from build123d import *

# Parameters (mm, degrees)
BOSS_EXTRU_1_DEPTH      = 20
CONG_1_R                = 2.38125
ESQUISSE2_W             = 63.5
ESQUISSE2_H             = 35.56
BOSS_EXTRU_2_DEPTH      = 5.08
EMPREINTE1_START        = -25.08
EMPREINTE1_DEPTH        = 5.08
D_PLACER_START          = -25.08
D_PLACER_LA_FACE1_DEPTH = 5.08
EMPREINTE4_START        = 17.46
EMPREINTE4_DEPTH        = 2.54
D_PLACER_START_2        = 16.952
D_PLACER_LA_FACE2_DEPTH = 3.048
CHANFREIN1_SIZE         = 6.35
CHANFREIN1_SIZE2        = 3.81
CHANFREIN2_SIZE         = 3.81
CHANFREIN2_SIZE2        = 6.35
BOSS_EXTRU_3_DEPTH      = 45.08
ESQUISSE4_W             = 44.45
ESQUISSE4_H             = 27.94
ENL_V_MAT_EXTRU_1_DEPTH = 38.1
ESQUISSE5_W             = 12.7
ESQUISSE5_H             = 3.81
BOSS_EXTRU_4_DEPTH      = 12.7
CONG_2_R                = 2.54
D_GAGEMENT_61_D         = 3.7973
ENL_V_MAT_EXTRU_2_DEPTH = 38.1
D_GAGEMENT_62_D         = 3.7973
D_GAGEMENT_62_DEPTH     = 18.796
D_GAGEMENT_62_TIP       = 1.140824014


# Read off the part's stored shape, not the designer's step: Empreinte1, Déplacer la face1, Empreinte4, Déplacer la face2
with BuildPart() as part:
    # Esquisse1 → Boss.-Extru.1 (new, symmetric)
    with BuildSketch(Plane.XY):
        Polygon((-31.75, -1.905), (-31.75, 33.655), (31.75, 33.655), (31.75, -1.905), (12.92225, -1.905), (12.92225, 4.445), (13.87475, 5.3975), (21.59, 5.3975), (21.59, 21.59), (-21.59, 21.59), (-21.59, 5.3975), (-13.87475, 5.3975), (-12.92225, 4.445), (-12.92225, -1.905), align=None)
    extrude(amount=BOSS_EXTRU_1_DEPTH, both=True)

    # Congé1
    cong_1_edges = [part.edges().sort_by_distance(p)[0] for p in [
        (21.59, 5.3975, 0),
        (21.59, 21.59, 0),
        (-21.59, 21.59, 0),
        (-21.59, 5.3975, 0),
    ]]
    fillet(cong_1_edges, radius=CONG_1_R)

    # Esquisse2 → Boss.-Extru.2 (add)
    with BuildSketch(Plane(origin=(0, 0, -20), x_dir=(-1, 0, 0), z_dir=(0, 0, -1))):
        with Locations((0, 15.875)):
            Rectangle(ESQUISSE2_W, ESQUISSE2_H)
    extrude(amount=BOSS_EXTRU_2_DEPTH)

    # Empreinte1 outline → Empreinte1 (cut)
    with BuildSketch(Plane.XY.offset(EMPREINTE1_START)):
        with BuildLine():
            Line((14.44625, 7.9375), (16.66875, 7.9375))
            ThreePointArc((16.66875, 7.9375), (17.366201977, 9.621298023), (19.05, 10.31875))
            Line((19.05, 10.31875), (19.05, 16.66875))
            ThreePointArc((19.05, 16.66875), (17.366201977, 17.366201977), (16.66875, 19.05))
            Line((16.66875, 19.05), (-16.66875, 19.05))
            ThreePointArc((-16.66875, 19.05), (-17.366201977, 17.366201977), (-19.05, 16.66875))
            Line((-19.05, 16.66875), (-19.05, 10.31875))
            ThreePointArc((-19.05, 10.31875), (-17.366201977, 9.621298023), (-16.66875, 7.9375))
            Line((-16.66875, 7.9375), (-14.44625, 7.9375))
            Line((-14.44625, 7.9375), (-11.90625, 5.3975))
            Line((-11.90625, 5.3975), (-11.90625, -1.905))
            Line((-11.90625, -1.905), (11.90625, -1.905))
            Line((11.90625, -1.905), (11.90625, 5.3975))
            Line((11.90625, 5.3975), (14.44625, 7.9375))
        make_face()
    extrude(amount=EMPREINTE1_DEPTH, mode=Mode.SUBTRACT)

    # Déplacer la face1 outline → Déplacer la face1 (cut)
    with BuildSketch(Plane.XY.offset(D_PLACER_START)):
        with BuildLine():
            Line((-14.867090979, 6.9215), (-12.92225, 4.976659021))
            Line((-12.92225, 4.976659021), (-12.92225, -1.905))
            Line((-12.92225, -1.905), (-11.90625, -1.905))
            Line((-11.90625, -1.905), (-11.90625, 5.3975))
            Line((-11.90625, 5.3975), (-14.44625, 7.9375))
            Line((-14.44625, 7.9375), (-16.66875, 7.9375))
            ThreePointArc((-16.66875, 7.9375), (-17.366201977, 9.621298023), (-19.05, 10.31875))
            Line((-19.05, 10.31875), (-19.05, 16.66875))
            ThreePointArc((-19.05, 16.66875), (-17.366201977, 17.366201977), (-16.66875, 19.05))
            Line((-16.66875, 19.05), (16.66875, 19.05))
            ThreePointArc((16.66875, 19.05), (17.366201977, 17.366201977), (19.05, 16.66875))
            Line((19.05, 16.66875), (19.05, 10.31875))
            ThreePointArc((19.05, 10.31875), (17.366201977, 9.621298023), (16.66875, 7.9375))
            Line((16.66875, 7.9375), (14.44625, 7.9375))
            Line((14.44625, 7.9375), (11.90625, 5.3975))
            Line((11.90625, 5.3975), (11.90625, -1.905))
            Line((11.90625, -1.905), (12.92225, -1.905))
            Line((12.92225, -1.905), (12.92225, 4.976659021))
            Line((12.92225, 4.976659021), (14.867090979, 6.9215))
            Line((14.867090979, 6.9215), (18.13805068, 6.9215))
            ThreePointArc((18.13805068, 6.9215), (18.084622467, 8.902877533), (20.066, 8.84944932))
            Line((20.066, 8.84944932), (20.066, 18.13805068))
            ThreePointArc((20.066, 18.13805068), (18.084622467, 18.084622467), (18.13805068, 20.066))
            Line((18.13805068, 20.066), (-18.13805068, 20.066))
            ThreePointArc((-18.13805068, 20.066), (-18.084622467, 18.084622467), (-20.066, 18.13805068))
            Line((-20.066, 18.13805068), (-20.066, 8.84944932))
            ThreePointArc((-20.066, 8.84944932), (-18.084622467, 8.902877533), (-18.13805068, 6.9215))
            Line((-18.13805068, 6.9215), (-14.867090979, 6.9215))
        make_face()
    extrude(amount=D_PLACER_LA_FACE1_DEPTH, mode=Mode.SUBTRACT)

    # Empreinte4 outline → Empreinte4 (cut)
    with BuildSketch(Plane.XY.offset(EMPREINTE4_START)):
        with BuildLine():
            ThreePointArc((-27.94, 7.62), (-26.67, 6.35), (-25.4, 7.62))
            Line((-25.4, 7.62), (-25.4, 20.32))
            ThreePointArc((-25.4, 20.32), (-26.67, 21.59), (-27.94, 20.32))
            Line((-27.94, 20.32), (-27.94, 7.62))
        make_face()
        with BuildLine():
            Line((25.4, 20.32), (25.4, 7.62))
            ThreePointArc((25.4, 7.62), (26.67, 6.35), (27.94, 7.62))
            Line((27.94, 7.62), (27.94, 20.32))
            ThreePointArc((27.94, 20.32), (26.67, 21.59), (25.4, 20.32))
        make_face()
    extrude(amount=EMPREINTE4_DEPTH, mode=Mode.SUBTRACT)

    # Déplacer la face2 outline → Déplacer la face2 (cut)
    with BuildSketch(Plane.XY.offset(D_PLACER_START_2)):
        with BuildLine():
            ThreePointArc((-28.448, 7.62), (-26.67, 5.842), (-24.892, 7.62))
            Line((-24.892, 7.62), (-24.892, 20.32))
            ThreePointArc((-24.892, 20.32), (-26.67, 22.098), (-28.448, 20.32))
            Line((-28.448, 20.32), (-28.448, 7.62))
        make_face()
        with BuildLine():
            Line((24.892, 20.32), (24.892, 7.62))
            ThreePointArc((24.892, 7.62), (26.67, 5.842), (28.448, 7.62))
            Line((28.448, 7.62), (28.448, 20.32))
            ThreePointArc((28.448, 20.32), (26.67, 22.098), (24.892, 20.32))
        make_face()
    extrude(amount=D_PLACER_LA_FACE2_DEPTH, mode=Mode.SUBTRACT)

    # Chanfrein1
    chanfrein1_edges = [part.edges().sort_by_distance(p)[0] for p in [
        (-12.92225, -1.905, -2.54),
    ]]
    chanfrein1_side = [part.faces().sort_by_distance(p)[0] for p in [
        (-22.336125, -1.905, -2.54),
    ]]
    chamfer(chanfrein1_edges, length=CHANFREIN1_SIZE, length2=CHANFREIN1_SIZE2, reference=chanfrein1_side[0])

    # Chanfrein2
    chanfrein2_edges = [part.edges().sort_by_distance(p)[0] for p in [
        (12.92225, -1.905, -2.54),
    ]]
    chanfrein2_side = [part.faces().sort_by_distance(p)[0] for p in [
        (12.92225, 1.302160596, -2.726935132),
    ]]
    chamfer(chanfrein2_edges, length=CHANFREIN2_SIZE, length2=CHANFREIN2_SIZE2, reference=chanfrein2_side[0])

    # Esquisse3 → Boss.-Extru.3 (add)
    with BuildSketch(Plane.XY.offset(20)):
        Polygon((-31.75, -1.905), (-31.75, -59.055), (31.75, -59.055), (31.75, -1.905), (22.225, -1.905), (22.225, -24.765), (-22.225, -24.765), (-22.225, -1.905), align=None)
    extrude(amount=-BOSS_EXTRU_3_DEPTH)

    # Esquisse4 → Enlèv. mat.-Extru.1 (cut)
    with BuildSketch(Plane.XY.offset(20)):
        with Locations((0, -38.735)):
            Rectangle(ESQUISSE4_W, ESQUISSE4_H)
    extrude(amount=-ENL_V_MAT_EXTRU_1_DEPTH, mode=Mode.SUBTRACT)

    # Esquisse5 → Boss.-Extru.4 (add)
    with BuildSketch(Plane(origin=(0, 0, -25.08), x_dir=(-1, 0, 0), z_dir=(0, 0, -1))):
        with Locations((0, -54.522979854)):
            Rectangle(ESQUISSE5_W, ESQUISSE5_H)
    extrude(amount=BOSS_EXTRU_4_DEPTH)

    # Congé2
    cong_2_edges = [part.edges().sort_by_distance(p)[0] for p in [
        (6.35, -54.522979854, -37.78),
        (-6.35, -54.522979854, -37.78),
    ]]
    fillet(cong_2_edges, radius=CONG_2_R)

    # Dégagement #61 (through all)
    with Locations(Plane(origin=(0, -52.617979854, 0), x_dir=(1, 0, 0), z_dir=(0, 1, 0))):
        with Locations((0, 31.43)):
            Hole(D_GAGEMENT_61_D / 2)

    # Esquisse8 → Enlèv. mat.-Extru.2 (cut)
    with BuildSketch(Plane(origin=(0, 0, -25.08), x_dir=(-1, 0, 0), z_dir=(0, 0, -1))):
        Polygon((22.86, 33.655), (31.75, 33.655), (31.75, 24.765), (26.67, 24.765), (22.86, 28.575), align=None)
    enl_v_mat_extru_2 = extrude(amount=-ENL_V_MAT_EXTRU_2_DEPTH, mode=Mode.SUBTRACT)

    # Symétrie1: Enlèv. mat.-Extru.2 across plane
    add(enl_v_mat_extru_2.mirror(Plane(origin=(0, 0, 0), x_dir=(0, 0, 1), z_dir=(1, 0, 0))), mode=Mode.SUBTRACT)

    # Dégagement #62
    with Locations(Plane(origin=(0, 0, 13.02), x_dir=(-1, 0, 0), z_dir=(0, 0, -1))):
        with Locations((27.94, 29.845), (-27.94, 29.845)):
            Hole(D_GAGEMENT_62_D / 2, depth=D_GAGEMENT_62_DEPTH)
            with Locations((0, 0, -(D_GAGEMENT_62_DEPTH + D_GAGEMENT_62_TIP / 2))):  # 118° drill point
                Cone(0, D_GAGEMENT_62_D / 2, D_GAGEMENT_62_TIP, mode=Mode.SUBTRACT)


solid = part.part
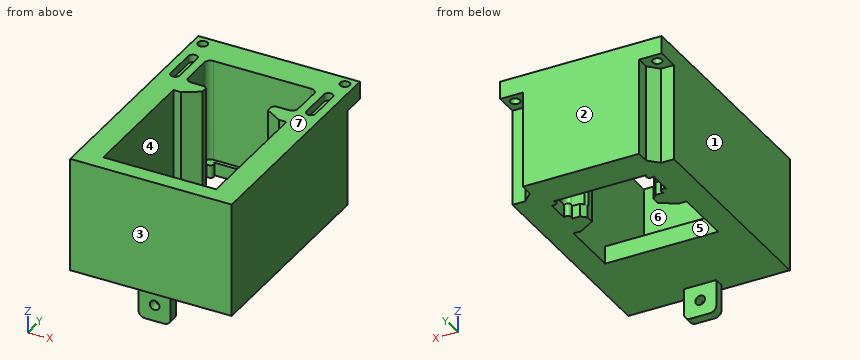
CAD build for the part. Positions are in the model's coordinates, mm. Face numbers are marked on the shaded views. A direction names the side the tool comes from. Coordinates: 2 decimals unless noted, no trailing zeros. Write each loop counter-clockwise with the first axis right and the second up, starting at its lowest first coordinate (ties: lowest second). Pieces come first, ordered by that corner, then holes. Notation, with made-up numbers: M 17.5,17 L 75.5,17 A8 cw 75.5,21 Z; hole C 85,84.5 d5. An arc over 180 degrees is marked long. Answer as a JSON object with one key per item and string values. Group by question number.
1) Mould opens along Y. For the marked faces 1, 2, 3 and 4 say: +Y half, -Y half, draft (parallel to the pull), parting line (faces both ways), or undercut.
2) Saw through at D-D (y = -29). Write the cut outline in (x, z) (3 decimals), plus the area to 3 significant figures.
3) Pin check, flat tips, straight feed: pin 1 Ø1.5 at (x, y) = (-5, -49.5) entering from -Z; pin 2 Ø4 at (x, z) = (1, -32.5) entering from +Y; pin 3 Ø14 at (x, z) = (0.5, -34.5) entering from -Y. Stop position of each tip, or through.
4) Saw through at B-B (y = -7). Write the cut outline in (x, z) (3 decimals).
5) Tool access for the marked faces 5, 6 and 7: list every direction of +Z, -Z, +X, -X, +Y, -Y with a clear straight run to the whole face (end or side of a thin tool).
6) Saw through at A-A (x = 0). Write the cut outline in (y, z) (3 decimals).
7) Wall check: line 1 (Y direction, x = -27.94, z = 18.5) (3 decimals); line 2 (X direction, y = -37, z = -12) (3 decimals); line 3 (Y direction, x = -2, z = 11) (3 decimals). Give the ranges that are in metal, low to high. Write a range as from..to.
Values follow:
{
 "1": {"face 1": "draft", "face 2": "+Y half", "face 3": "-Y half", "face 4": "undercut"},
 "2": {"outline": "M -31.75,-25.08 L 31.75,-25.08 L 31.75,20 L 22.225,20 L 22.225,-18.1 L -22.225,-18.1 L -22.225,20 L -31.75,20 Z", "area": "1,170 mm2"},
 "3": {"pin 1": "stops at z = -25.08", "pin 2": "stops at y = -52.62", "pin 3": "stops at y = -56.43"},
 "4": {"outline": "M -31.75,-25.08 L -22.225,-25.08 L -22.225,20 L -31.75,20 Z; M 22.225,-25.08 L 31.75,-25.08 L 31.75,20 L 22.225,20 Z"},
 "5": {"face 5": "+Z, -Z", "face 6": "+Z", "face 7": "+Z, +X, -X, +Y, -Y"},
 "6": {"outline": "M -59.055,-25.08 L -56.428,-25.08 L -56.428,-29.531 L -52.618,-29.531 L -52.618,-25.08 L -24.765,-25.08 L -24.765,-18.1 L -52.705,-18.1 L -52.705,20 L -59.055,20 Z; M -56.428,-37.78 L -52.618,-37.78 L -52.618,-33.329 L -56.428,-33.329 Z; M 20.066,-25.08 L 33.655,-25.08 L 33.655,20 L 21.59,20 L 21.59,-20 L 20.066,-20 Z"},
 "7": {"line 1": "y = -59.055..6.376, 21.564..27.946, 31.744..33.655", "line 2": "x = -31.75..-22.225, 22.225..31.75", "line 3": "y = -59.055..-52.705, 21.59..33.655"}
}
